The listing builds one solid part. Answer for the finished solid, in the listing's coordinates (mm). Face numbers are marked on the shaded views. A direction names the side the tool comes from. Give positions to 0.01 mm unless a question says otherwise; leave off trailing zeros. Order: outer loops, then holes, each group sorted by start corner. A loop starts at its lowest first (then second) coordinate and runs counter-clockwise, first axis right, second up. Notation, with made-up numbers: (56.25, 52.25) - (76.25, 52.25) arc R17 ccw to (76.25, 58.25) - close; hole circle Ø9 at (84.25, -33). An arc over 180 degrees is marked (long way). Answer as a JSON object with one key per item and string values. Group by question number.
Q1. A cutting plane is placed at A-A, the plane y = 20. Give the vertices of the cut face in (x, z), and give its area (3 significant figures).
Q2. Consider line 1 (Y direction, x = 9.25, z = 35); line 2 (X direction, y = 56, z = 0); line 3 (Z direction, x = 29.5, y = 52.5). Determine where each line is inside the solid, lowest interval first.
Q3. The mould has two halves that part along X. Classify the marked faces 4, 5 and 6: released by +X, released by -X, zero draft, split by the parting line, or undercut.
Q4. A cutting plane is placed at D-D, the plane x = 15. Give the vertices of the cut face in (y, z), and give its area (3 significant figures).
Q5. For the marked faces 1, 2 and 3, determine the directions among +Z, -Z, +X, -X, +Y, -Y from which every point of the face is accessible in a straight line to the end or side of a thin tool.
Q6. Given pin 1 (2 mm diameter, centred on x = 30, y = 35.5, fed in from +Z); pin 2 (9 mm diameter, centred on y = 33.5, z = 35, fed in from +X), each flat-ended and moving along its own axis, determine where each tip first touches the part or whether it passes through.
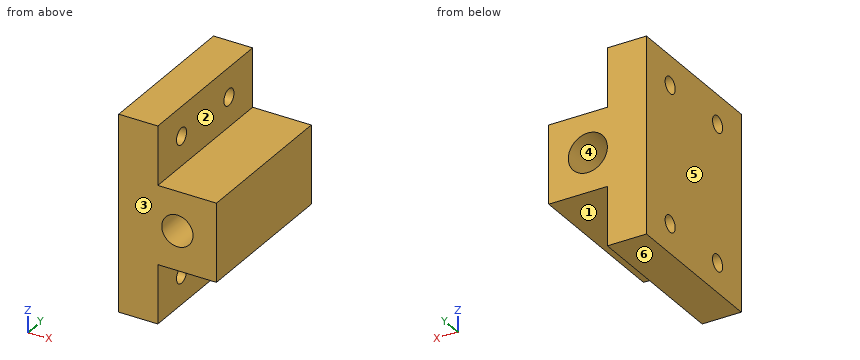
from build123d import *

# Parameters (mm, degrees)
SKETCH1_W           = 50
SKETCH1_H           = 40
BOSS_EXTRUDE1_DEPTH = 80
SKETCH4_W           = 100
SKETCH4_H           = 80
BOSS_EXTRUDE2_DEPTH = 20
SKETCH5_R           = 4.24
SCREW_HOLE_DEPTH    = 99.994949366
SKETCH6_R           = 8
ROD_HOLE_DEPTH      = 107.77078252
SKETCH7_R           = 10
CUT_EXTRUDE5_DEPTH  = 50
CHAMFER2_SIZE       = 2


with BuildPart() as part:
    # Sketch1 → Boss-Extrude1 (new body)
    with BuildSketch(Plane(origin=(0, 0, 0), x_dir=(1, 0, 0), z_dir=(0, 1, 0))):
        with Locations((25, 0)):
            Rectangle(SKETCH1_W, SKETCH1_H)
    extrude(amount=BOSS_EXTRUDE1_DEPTH)

    # Sketch4 → Boss-Extrude2 (add)
    with BuildSketch(Plane.ZY):
        with Locations((0, 40)):
            Rectangle(SKETCH4_W, SKETCH4_H)
    extrude(amount=-BOSS_EXTRUDE2_DEPTH)

    # Sketch5 → screw hole (cut, through all)
    with BuildSketch(Plane(origin=(20, 0, 0), x_dir=(0, 0, -1), z_dir=(1, 0, 0))):
        with Locations((-35, 20)):
            Circle(SKETCH5_R)
        with Locations((-35, 60)):
            Circle(SKETCH5_R)
    screw_hole = extrude(amount=-SCREW_HOLE_DEPTH, mode=Mode.SUBTRACT)

    # Mirror1: screw hole across plane
    add(screw_hole.mirror(Plane.XY), mode=Mode.SUBTRACT)

    # Sketch6 → rod hole (cut, through all)
    with BuildSketch(Plane(origin=(0, 80, 0), x_dir=(1, 0, 0), z_dir=(0, 1, 0))):
        with Locations(Location((30, 0, 0), (0, 0, 270))):
            Circle(SKETCH6_R)
    extrude(amount=-ROD_HOLE_DEPTH, mode=Mode.SUBTRACT)

    # Sketch7 → Cut-Extrude5 (cut)
    with BuildSketch(Plane(origin=(0, 80, 0), x_dir=(1, 0, 0), z_dir=(0, 1, 0))):
        with Locations(Location((30, 0, 0), (0, 0, 270))):
            Circle(SKETCH7_R)
    extrude(amount=-CUT_EXTRUDE5_DEPTH, mode=Mode.SUBTRACT)

    # Chamfer2
    chamfer2_edges = [part.edges().sort_by_distance(p)[0] for p in [
        (30, 30, -8),
    ]]
    chamfer(chamfer2_edges, length=CHAMFER2_SIZE - 0.0001)  # a hair under: the kernel refuses the full size


solid = part.part
Reply:
{
 "1": {"outline": "(0, -50) - (20, -50) - (20, -39.24) - (0, -39.24) - close; (0, -30.76) - (20, -30.76) - (20, -20) - (50, -20) - (50, 20) - (20, 20) - (20, 30.76) - (0, 30.76) - close; (0, 39.24) - (20, 39.24) - (20, 50) - (0, 50) - close; hole circle Ø16 at (30, 0)", "area": "2,660 mm^2"},
 "2": {"line 1": "y = 0 to 15.76, 24.24 to 55.76, 64.24 to 80", "line 2": "x = 0 to 20, 40 to 50", "line 3": "z = -20 to -9.99, 9.99 to 20"},
 "3": {"face 4": "undercut", "face 5": "released by -X", "face 6": "zero draft"},
 "4": {"outline": "(0, -50) - (80, -50) - (80, 50) - (0, 50) - close; hole circle Ø8.48 at (20, -35); hole circle Ø8.48 at (20, 35); hole circle Ø8.48 at (60, -35); hole circle Ø8.48 at (60, 35)", "area": "7,770 mm^2"},
 "5": {"face 1": "-Z, +X, +Y, -Y", "face 2": "+Z, +X, +Y, -Y", "face 3": "+Z, -Z, +X, -X, -Y"},
 "6": {"pin 1": "stops at z = 20", "pin 2": "stops at x = 20"}
}
